Part print with two shaded views. Sizes in mm from the minimum x, y, z corner. Round coordinates to 2 decimals unless told otherwise and drop trailing zeros. Loops run counter-clockwise (first coordinate to the right, second up) from the corner with the lowest first, then second, coordinate; pieces in that order, holes last. Notation, with made-up numbers: (-37, 58.25) -> (-32, 58.25) arc R19 cw to (-32, 64.25) -> close; hole circle Ø5 at (68, 23.5). An arc over 180 degrees is marked (long way). Use a Markdown table: item, result. Add a question column.
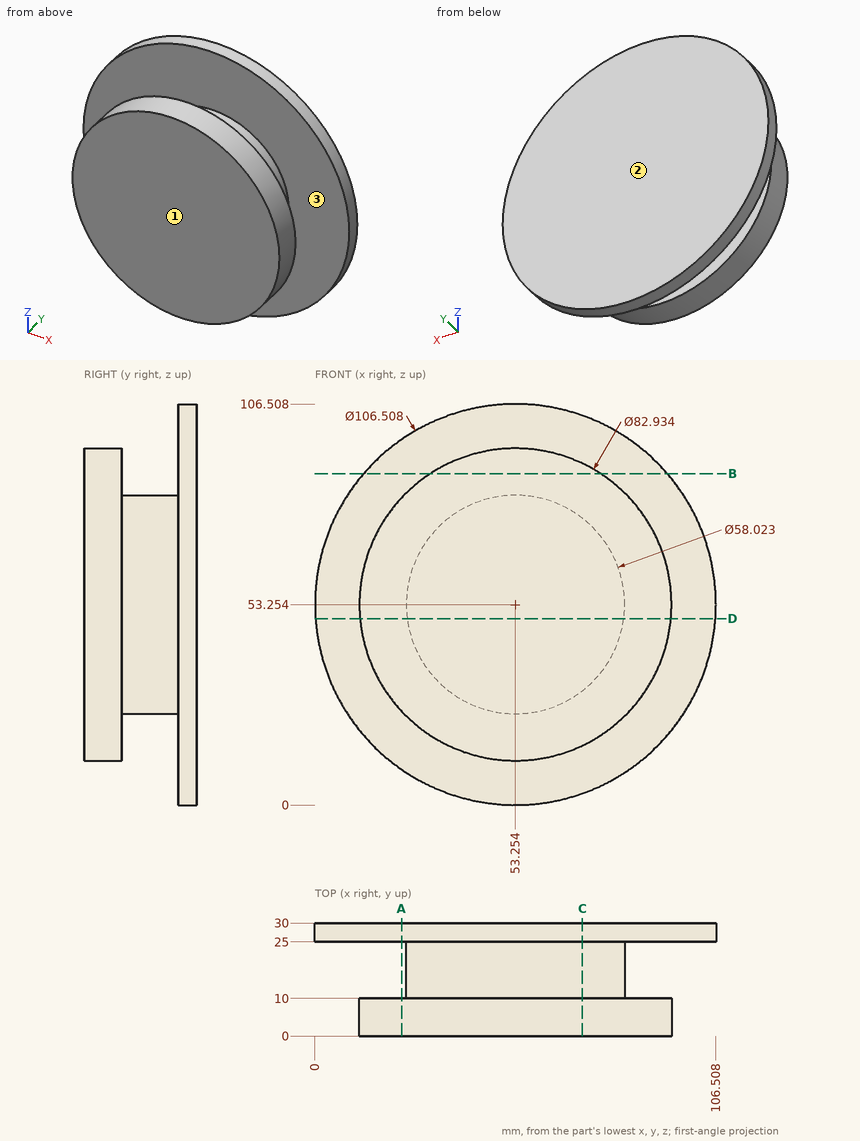
1) Pull direction Y, two halves, no side cores. Call the marked faces 1, 2 and 3: +Y half, -Y half, draft (parallel to the pull), parting line (faces both ways), or undercut.
2) Cut at A-A on x = 23. Write the cut outline in (y, z), and give its area (3 significant figures).
3) Cut at D-D on z = 49.5. Write the cut outline in (x, y), and give its area (3 significant figures).
4) Cut at C-C on x = 71. Write the cut outline in (y, z) (1 decimal), and give its area (3 significant figures).
5) Wall check: probe 1 along Y at (x, z) = (25, 42); probe 2 along Y at (x, z) = (11, 42.5); probe 3 along Z at (x, y) = (14, 26.75) (1 decimal). Give the ranges that are in metal, low to high. Write a range as from..to.
6) Cut at B-B on z = 88. Write the cut outline in (x, y), and give its area (3 significant figures).
7) Pin check, flat tips, straight feed: pin 1 Ø1.5 at (y, z) = (8, 81.5) entering from +X (1 decimal); pin 2 Ø1.5 at (x, z) = (77, 50.5) entering from -Y; pin 3 Ø1.5 at (y, z) = (19, 73) entering from +X; pin 4 Ø12 at (x, y) = (49.5, 15.5) entering from +Z. Stop position of each tip, or through.
Established:
| question | item | result |
|---|---|---|
| 1 | face 1 | -Y half |
| 1 | face 2 | +Y half |
| 1 | face 3 | undercut |
| 2 | outline | (0, 24.9) -> (10, 24.9) -> (10, 81.61) -> (0, 81.61) -> close; (25, 9.43) -> (30, 9.43) -> (30, 97.08) -> (25, 97.08) -> close |
| 2 | area | 1,010 mm^2 |
| 3 | outline | (0.13, 25) -> (24.49, 25) -> (24.49, 10) -> (11.96, 10) -> (11.96, 0) -> (94.55, 0) -> (94.55, 10) -> (82.02, 10) -> (82.02, 25) -> (106.38, 25) -> (106.38, 30) -> (0.13, 30) -> close |
| 3 | area | 2,220 mm^2 |
| 4 | outline | (0, 15.8) -> (10, 15.8) -> (10, 30.3) -> (25, 30.3) -> (25, 3) -> (30, 3) -> (30, 103.5) -> (25, 103.5) -> (25, 76.2) -> (10, 76.2) -> (10, 90.7) -> (0, 90.7) -> close |
| 4 | area | 1,940 mm^2 |
| 5 | probe 1 | y = 0..10, 25..30 |
| 5 | probe 2 | y = 25..30 |
| 5 | probe 3 | z = 17.3..89.2 |
| 6 | outline | (12.9, 25) -> (93.61, 25) -> (93.61, 30) -> (12.9, 30) -> close; (30.62, 0) -> (75.89, 0) -> (75.89, 10) -> (30.62, 10) -> close |
| 6 | area | 856 mm^2 |
| 7 | pin 1 | stops at x = 84.3 |
| 7 | pin 2 | stops at y = 0 |
| 7 | pin 3 | stops at x = 75.18 |
| 7 | pin 4 | stops at z = 94.7 |
